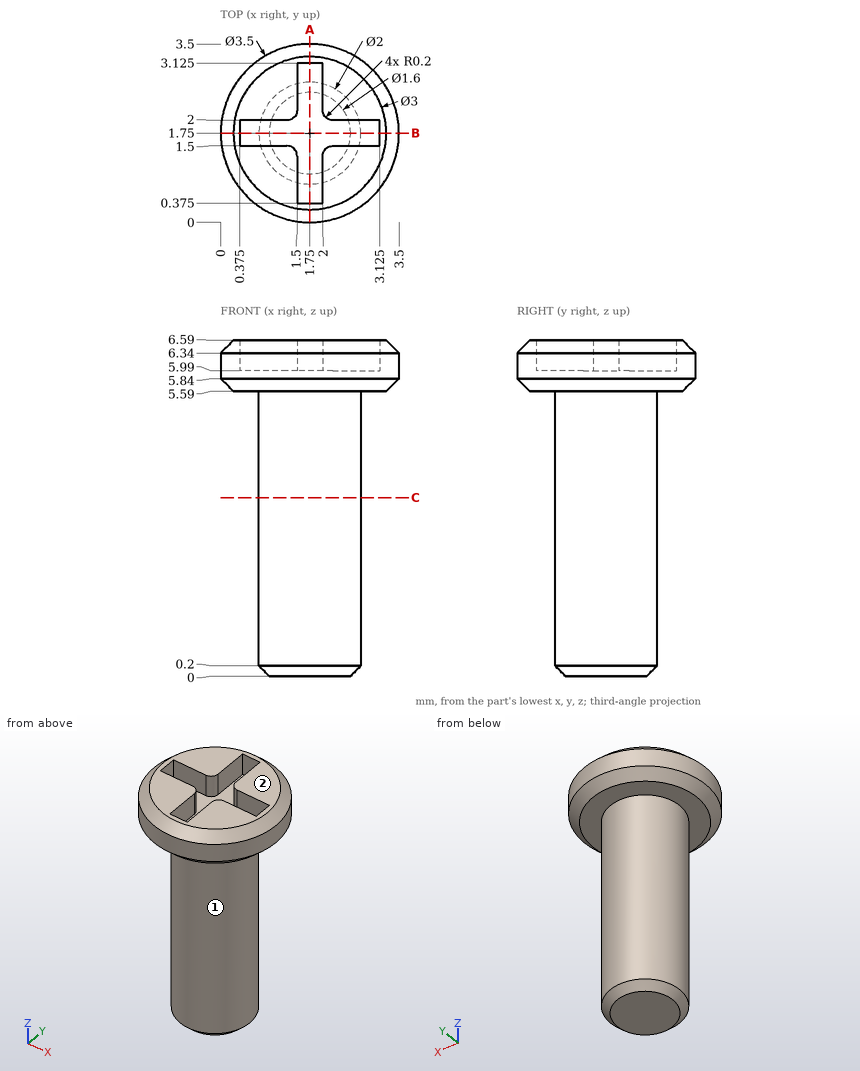
Design review of the part shown in the three views and the two pictorial views. Dimensions are in mm from the part's minimum x, y and z. A direction names the side the tool comes from. Coordinates: 2 decimals unless noted, no trailing zeros. Order: outer loops, then holes, each group sorted by start corner. A loop starts at its lowest first (then second) coordinate and runs counter-clockwise, first axis right, second up.
1) For the marked faces 1 and 2, list the 3-axis set-ups (+Z, -Z, +X, -X, +Y, -Y) from which the entire face can be reached by the end or side of a thin tool; tool diameter is ignored.
2) Wall thickness on line 1 along X through (y, z) = (2.55, 6.25); line 2 along Z through (x, y) = (3.05, 1.85); line 3 along Y through (x, z) = (1.7, 3.5): over which ranges is each line inside the solid? List them lowest first.
3) Clearance check with flat-ended pins moving along their axes: pin 1 (0.5 mm diameter, centred on x = 1, z = 6, fed in from +Y); pin 2 (1 mm diameter, centred on y = 1, z = 6, fed in from +X); pin 3 (1.5 mm diameter, centred on x = 2.5, z = 3, fed in from -Y). State where each tip first meets the part, or that it passes through.
4) Take a section at A-A, the plane x = 1.75. Give the boundary of the cut face in (y, z) (3 decimals), and give its area (3 significant figures).
5) Take a section at C-C, the plane z = 3.5. Give the boundary of the cut face in (x, y).
Returned:
1. face 1: -Z
1. face 2: +Z, +X, -X, +Y, -Y
2. line 1: x = 0.19 to 1.5, 2 to 3.31
2. line 2: z = 5.59 to 5.99
2. line 3: y = 0.75 to 2.75
3. pin 1: stops at y = 3.43
3. pin 2: stops at x = 3.48
3. pin 3: stops at y = 0.75
4. outline: (0, 5.84) - (0.25, 5.59) - (0.75, 5.59) - (0.75, 0.2) - (0.95, 0) - (2.55, 0) - (2.75, 0.2) - (2.75, 5.59) - (3.25, 5.59) - (3.5, 5.84) - (3.5, 6.34) - (3.25, 6.59) - (3.125, 6.59) - (3.125, 5.99) - (0.375, 5.99) - (0.375, 6.59) - (0.25, 6.59) - (0, 6.34) - close
4. area: 12.9 mm2
5. outline: circle Ø2 at (1.75, 1.75)
